Could you check a few things on this model? Use its own coordinates, in mm. Face numbers are marked on the shaded views. A direction names the side the tool comes from. Coordinates: 2 decimals unless noted, no trailing zeros. Loops run counter-clockwise (first coordinate to the right, second up) from the corner with the lowest first, then second, coordinate; pieces in that order, holes last. Notation, with made-up numbers: (72.5, 50.5) - (114.5, 50.5) arc R32 ccw to (114.5, 84.5) - close; hole circle Ø11 at (78, -28). An arc over 180 degrees is marked (long way). One line per item, written item: value. Start each with the question number.
(1) If I drill on line 1 along Y through (x, z) = (-52, 51), over which ranges is the centre line in solid material (lowest first)? Write a range as from..to.
(2) If we section it at A-A on x = -78.5: Write out the boundary of the cut face in (y, z).
(3) If we section it at B-B on z = 44: Write out the boundary of the cut face in (x, y), then the cut area to 3 significant figures.
(4) On a 3-axis mill with a long thin cutter (end or side, diameter ignored), from which of +Z, -Z, +X, -X, +Y, -Y can I reach the whole of each face in a straight line? I mean the marked faces 1, 2 and 3. Say none if no direction works.
(5) I'm going to push flat-ended pins straight in: P1, Ø5.5, axis at x = -23.5, y = -76, coming from the +Z side; P2, Ø18, axis at x = -10.5, z = 47, coming from the +Y side. Where does each tip first touch, or does it pass through?
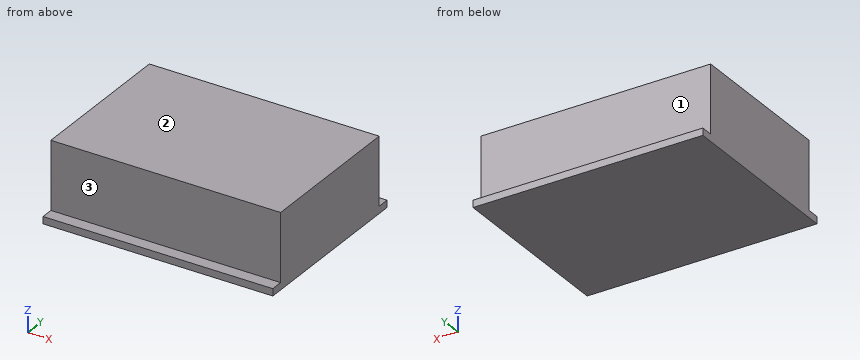
```python
from build123d import *

# Parameters (mm, degrees)
F0_W     = 205
F0_H     = 138
F1_DEPTH = 67
F2_W     = 205
F2_H     = 6.35
F3_DEPTH = 11


# Not quite as in the source:
# - a pattern or mirror of a feature is missing from the dataset's text; its kind, count and spacing are read off the source's solid


with BuildPart() as f1:
    # F0 (on Top) → F1 (new body)
    with BuildSketch(Plane.XY):
        Rectangle(F0_W, F0_H)
    extrude(amount=F1_DEPTH)

    # F2 (on face) → F3 (join)
    with BuildSketch(Plane.XZ.offset(69)):
        with Locations((0, 3.175)):
            Rectangle(F2_W, F2_H)
    f3 = extrude(amount=F3_DEPTH)

    # F3_copies: F3 across plane
    add(f3.mirror(Plane.ZX))


solid = f1.part
```
Values:
1. line 1: y = -69..69
2. outline: (-80, 0) - (80, 0) - (80, 6.35) - (69, 6.35) - (69, 67) - (-69, 67) - (-69, 6.35) - (-80, 6.35) - close
3. outline: (-102.5, -69) - (102.5, -69) - (102.5, 69) - (-102.5, 69) - close
3. area: 28,300 mm2
4. face 1: +Z, +X, -X, +Y
4. face 2: +Z, +X, -X, +Y, -Y
4. face 3: +Z, +X, -X, -Y
5. P1: stops at z = 6.35
5. P2: stops at y = 69
